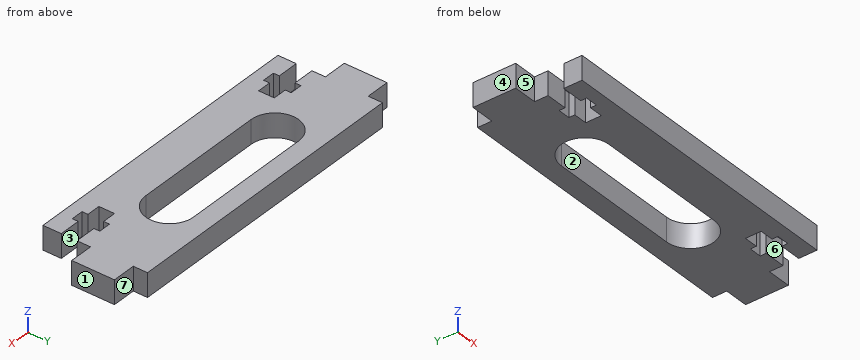
```python
from build123d import *

# Parameters (mm, degrees)
PLASTINA_DEPTH = 5


with BuildPart() as part:
    # Eskiz_kontur → Plastina (new body)
    with BuildSketch(Plane.XY):
        Polygon((32.5, 12), (27.5, 12), (27.5, 9.15), (23, 9.15), (23, 10.4), (20.4, 10.4), (20.4, 9.15), (17.5, 9.15), (17.5, 5.85), (20.4, 5.85), (20.4, 4.6), (23, 4.6), (23, 5.85), (27.5, 5.85), (27.5, 2), (-35, 2), (-35, 5.85), (-30.5, 5.85), (-30.5, 4.6), (-27.9, 4.6), (-27.9, 5.85), (-25, 5.85), (-25, 9.15), (-27.9, 9.15), (-27.9, 10.4), (-30.5, 10.4), (-30.5, 9.15), (-35, 9.15), (-35, 12), (-40, 12), (-40, 21), (-35, 21), (-35, 24), (27.5, 24), (27.5, 21), (32.5, 21), align=None)
        with BuildLine():
            Line((10.25, 20), (-17.75, 20))
            ThreePointArc((-17.75, 20), (-22.75, 15), (-17.75, 10))
            Line((-17.75, 10), (10.25, 10))
            ThreePointArc((10.25, 10), (15.25, 15), (10.25, 20))
        make_face(mode=Mode.SUBTRACT)
    extrude(amount=PLASTINA_DEPTH)


solid = part.part
```
Source: CAD feature listing. Evaluate the final solid. Frame: model axes, mm. Face numbers are marked on the shaded views. A direction names the side the tool comes from. Round coordinates to 2 decimals unless told otherwise and drop trailing zeros. Loops run counter-clockwise (first coordinate to the right, second up) from the corner with the lowest first, then second, coordinate; pieces in that order, holes last.
1. Contact query for flat-ended pins moving along their axis: pin 1 (0.6 mm diameter, centred on y = 5.5, z = 2, fed in from -X); pin 2 (2.5 mm diameter, centred on x = 29, z = 1.5, fed in from +Y); pin 3 (8 mm diameter, centred on x = 2.5, y = 11.5, fed in from -Z); pin 4 (1.7 mm diameter, centred on y = 7, z = 3, fed in from +X). Output: stop coordinate, or through.
2. Section query A-A on x = -29.5. Output: boundary loops of the cut face in (y, z).
3. Section query B-B on y = 17.75. Output: boundary loops of the cut face in (x, z).
4. Ray query, L1, parallel to X at y = 5.5, z = 4; L2, parallel to Y at x = -17.5, z = 3.8; L3, parallel to Y at x = -26, z = 4.45. Return the intervals inside material, ascending.
5. Access query for the marked faces 5, 6 and 7. Directions: +Z, -Z, +X, -X, +Y, -Y. A direction counts if a zero-diameter tool reaches every point of the face in a straight line with its end or side. Return the directions, or none.
6. Mould query, pull axis X, two halves, no side actions, for the marked faces 1, 2, 3 and 4. Classes: released by +X, released by -X, zero draft, split by the parting line, or undercut.
Answers below:
1. pin 1: stops at x = -35
1. pin 2: stops at y = 21
1. pin 3: stops at z = 0
1. pin 4: stops at x = 17.5
2. outline: (2, 0) - (4.6, 0) - (4.6, 5) - (2, 5) - close; (10.4, 0) - (24, 0) - (24, 5) - (10.4, 5) - close
3. outline: (-40, 0) - (-21.93, 0) - (-21.93, 5) - (-40, 5) - close; (14.43, 0) - (32.5, 0) - (32.5, 5) - (14.43, 5) - close
4. L1: x = -35 to -30.5, -27.9 to 20.4, 23 to 27.5
4. L2: y = 2 to 10, 20 to 24
4. L3: y = 2 to 5.85, 9.15 to 24
5. face 5: +Z, -Z, -X, -Y
5. face 6: +Z, -Z, +X
5. face 7: +Z, -Z, +X, +Y
6. face 1: released by +X
6. face 2: undercut
6. face 3: zero draft
6. face 4: released by -X
